The listing builds one solid part. Answer for the finished solid, in the listing's coordinates (mm). A direction names the side the tool comes from. Coordinates: 2 decimals unless noted, no trailing zeros. Order: outer loops, then holes, each group sorted by start corner. A loop starts at its lowest first (then second) coordinate and runs counter-clockwise, first axis right, second up.
Autodesk Inventor part; units mm, degrees
ref_plane "YZ Plane" through (0, 0, 0) normal (1, 0, 0) x (0, 1, 0)
ref_plane "XZ Plane" through (0, 0, 0) normal (0, 1, 0) x (-1, 0, 0)
ref_plane "XY Plane" through (0, 0, 0) normal (0, 0, 1) x (1, 0, 0)
sketch "Sketch1" plane through (0, 0, 0) normal (0, 0, 1) x (1, 0, 0)
  line L0 (50, -70) -> (50, 25)
  line L1 (-50, 25) -> (-50, -70)
  line L2 (0, 0) -> (-38.1854, 57.2781) construction
  arc A0 (50, 25) -> (-50, 25) centre (0, 25) ccw
  line L3 (-45, -90) -> (45, -90)
  line L4 (0, 0) -> (38.1854, 57.2781) construction
  line L5 (50, -70) -> (50, -85)
  line L6 (-50, -70) -> (-50, -85)
  arc A1 (45, -90) -> (50, -85) centre (45, -85) ccw
  arc A2 (-50, -85) -> (-45, -90) centre (-45, -85) ccw
  line L7 (-47.25, 25) -> (-47.25, -70)
  line L8 (-47.25, -70) -> (-47.25, -85)
  arc A3 (-47.25, -85) -> (-45, -87.25) centre (-45, -85) ccw
  line L9 (-45, -87.25) -> (45, -87.25)
  arc A4 (45, -87.25) -> (47.25, -85) centre (45, -85) ccw
  line L10 (47.25, -85) -> (47.25, -70)
  line L11 (47.25, -70) -> (47.25, 25)
  arc A5 (47.25, 25) -> (-47.25, 25) centre (0, 25) ccw
  dimension "d0" = 5
  dimension "d1" = 2.75
extrude "Extrusion1" add sketch "Sketch1" along normal blind 2.5 contours L5 A1 L3 A2 L6 L1 A0 L0 | A5 L11 L10 A4 L9 A3 L8 L7
sketch "Sketch2" plane through (0, 0, 0) normal (0, 0, -1) x (-1, 0, 0)
  line L0 (50, -70) -> (50, 25)
  line L1 (-50, 25) -> (-50, -70)
  line L2 (0, 0) -> (-38.1854, 57.2781) construction
  arc A0 (50, 25) -> (-50, 25) centre (0, 25) ccw
  line L3 (-45, -90) -> (45, -90)
  line L4 (0, 0) -> (38.1854, 57.2781) construction
  line L5 (50, -70) -> (50, -85)
  line L6 (-50, -70) -> (-50, -85)
  arc A1 (45, -90) -> (50, -85) centre (45, -85) ccw
  arc A2 (-50, -85) -> (-45, -90) centre (-45, -85) ccw
  line L7 (-47.25, 25) -> (-47.25, -70)
  line L8 (-47.25, -70) -> (-47.25, -85)
  arc A3 (-47.25, -85) -> (-45, -87.25) centre (-45, -85) ccw
  line L9 (-45, -87.25) -> (45, -87.25)
  arc A4 (45, -87.25) -> (47.25, -85) centre (45, -85) ccw
  line L10 (47.25, -85) -> (47.25, -70)
  line L11 (47.25, -70) -> (47.25, 25)
  arc A5 (47.25, 25) -> (-47.25, 25) centre (0, 25) ccw
  line L12 (-45.25, 25) -> (-45.25, -70)
  line L13 (-45.25, -70) -> (-45.25, -85)
  arc A6 (-45.25, -85) -> (-45, -85.25) centre (-45, -85) ccw
  line L14 (-45, -85.25) -> (45, -85.25)
  arc A7 (45, -85.25) -> (45.25, -85) centre (45, -85) ccw
  line L15 (45.25, -85) -> (45.25, -70)
  line L16 (45.25, -70) -> (45.25, 25)
  arc A8 (45.25, 25) -> (-45.25, 25) centre (0, 25) ccw
  line L17 (-5, -80.25) -> (5, -80.25)
  line L18 (-5, -85.25) -> (-5, -80.25)
  line L19 (5, -80.25) -> (5, -85.25)
  line L20 (-5, 65.25) -> (5, 65.25)
  line L21 (-5, 69.9729) -> (-5, 65.25)
  line L22 (5, 65.25) -> (5, 69.9729)
  dimension "d4" = 5
  dimension "d5" = 2.75
  dimension "d6" = 2
extrude "Extrusion2" add sketch "Sketch2" along normal blind 5 contours A5 L11 L10 A4 L9 A3 L8 L7 | A8 L22 L20 L21 | L18 L17 L19 L14
sketch "Sketch3" plane through (-45, -87.25, 0) normal (0, -1, 0) x (1, 0, 0)
  line L0 (45, 0) -> (45, -5)
  line L1 (-2.25, -5) -> (92.25, -5)
  circle A0 centre (45, -2.5) radius 1.45
  line L2 (0, 0) -> (90, 0)
  dimension "d10" = 2.9
  dimension "d16" = 5
extrude "Extrusion3" cut sketch "Sketch3" against normal through all
sketch "Sketch4" plane through (0, 0, 0) normal (0, 0, -1) x (-1, 0, 0)
  arc A0 (-1.5, 38.5981) -> (1.5, 38.5981) centre (0, 36) ccw
  arc A1 (1.5, 40) -> (-1.5, 40) centre (0, 40) ccw
  line L0 (-1.5, 40) -> (-1.5, 38.5981)
  line L1 (1.5, 40) -> (1.5, 38.5981)
  point P0 (0, 0)
  dimension "d13" = 3
extrude "Extrusion4" cut sketch "Sketch4" against normal blind 10
properties part number "lid"
1) Each of these flat-tipped pins is pushed along its axis until it touches: P1, Ø1, axis at x = 11.5, y = 52.5, coming from the -Z side; P2, Ø0.7, axis at y = 39, z = 1, coming from the -X side; P3, Ø1.5, axis at x = 1.5, z = -2, coming from the -Y side; P4, Ø7, axis at x = 0, y = 36, coming from the +Z side. Where does it stop, or does it pass through?
2) A cutting plane is placed at C-C, the plane y = 36. Write down the section's boundary in (x, z) (3 decimals).
3) Straight lines are drawn through the part: probe 1 along X at (y, z) = (-84.5, -2.5); probe 2 along Y at (x, z) = (0, 0.85); probe 3 along X at (y, z) = (16.5, -0.25). For each, find the intervals that lie inside material, in ascending order.
4) A cutting plane is placed at A-A, the plane z = -2.5. Write down the section's boundary in (x, y).
5) The mould has two halves that part along X. Classify faces 1 (the cylindrical face through (-1.099, 74.988, 1.232)), 2 (the flat face through (25, -85.25, -2)), 3 (the flat face through (48, -1, 0)): released by +X, released by -X, zero draft, split by the parting line, or undercut.
6) A cutting plane is placed at B-B, the plane y = -68. Write down the section's boundary in (x, z), plus the area to 3 significant figures.
7) For faces 4 (the cylindrical face through (0, 33, 1)), 5 (the flat face through (-47.25, -31, -2)), 6 (the flat face through (-45.25, -31, -2)), determine the directions among +Z, -Z, +X, -X, +Y, -Y from which every point of the face is accessible in a straight line to the end or side of a thin tool.
8) A cutting plane is placed at D-D, the plane x = 27.5. Write down the section's boundary in (y, z).
Working result:
1. P1: stops at z = 0
1. P2: stops at x = -48.1
1. P3: stops at y = -87.25
1. P4: stops at z = 2.5
2. outline: (-48.775, 0) - (-45.952, 0) - (-45.952, -5) - (-43.893, -5) - (-43.893, 0) - (-3, 0) - (-3, 2.5) - (-48.775, 2.5) - close; (3, 0) - (43.893, 0) - (43.893, -5) - (45.952, -5) - (45.952, 0) - (48.775, 0) - (48.775, 2.5) - (3, 2.5) - close
3. probe 1: x = -47.25 to -45.25, -5 to -1.45, 1.45 to 5, 45.25 to 47.25
3. probe 2: y = -90 to 33, 41.5 to 75
3. probe 3: x = -47.25 to -45.25, 45.25 to 47.25
4. outline: (-47.25, -85) arc R2.25 ccw to (-45, -87.25) - (-1.45, -87.25) - (-1.45, -80.25) - (-5, -80.25) - (-5, -85.25) - (-45, -85.25) arc R0.25 cw to (-45.25, -85) - (-45.25, 25) arc R45.25 cw to (-5, 69.97) - (-5, 65.25) - (-1.45, 65.25) - (-1.45, 72.23) arc R47.25 ccw to (-47.25, 25) - close; (1.45, -87.25) - (45, -87.25) arc R2.25 ccw to (47.25, -85) - (47.25, 25) arc R47.25 ccw to (1.45, 72.23) - (1.45, 65.25) - (5, 65.25) - (5, 69.97) arc R45.25 cw to (45.25, 25) - (45.25, -85) arc R0.25 cw to (45, -85.25) - (5, -85.25) - (5, -80.25) - (1.45, -80.25) - close
5. face 1: split by the parting line
5. face 2: undercut
5. face 3: zero draft
6. outline: (-50, 0) - (-47.25, 0) - (-47.25, -5) - (-45.25, -5) - (-45.25, 0) - (45.25, 0) - (45.25, -5) - (47.25, -5) - (47.25, 0) - (50, 0) - (50, 2.5) - (-50, 2.5) - close
6. area: 270 mm2
7. face 4: +Z, -Z
7. face 5: -Z, -X, +Y, -Y
7. face 6: -Z
8. outline: (-90, 0) - (-87.25, 0) - (-87.25, -5) - (-85.25, -5) - (-85.25, 0) - (60.93, 0) - (60.93, -5) - (63.42, -5) - (63.42, 0) - (66.76, 0) - (66.76, 2.5) - (-90, 2.5) - close
